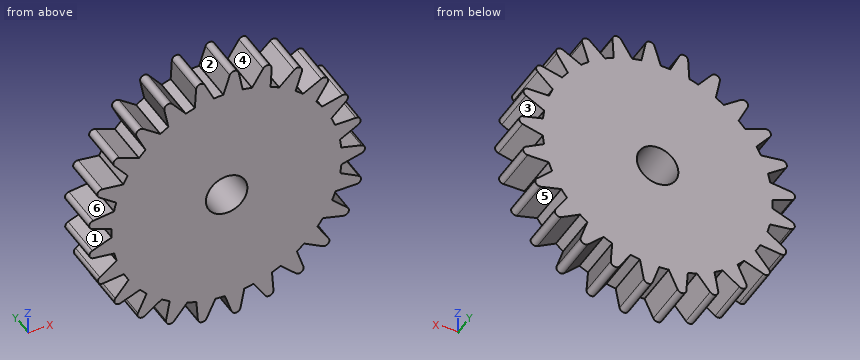
from build123d import *

# Parameters (mm, degrees)
BOSS_EXTRUDE1_DEPTH = 5
SKETCH6_R           = 2.25
CUT_EXTRUDE1_DEPTH  = 6


with BuildPart() as part:
    # Sketch1 → Boss-Extrude1 (new body)
    with BuildSketch(Plane(origin=(0, -74.1, 0), x_dir=(1, 0, 0), z_dir=(0, 1, 0))):
        with BuildLine():
            Line((-5.573417888, -7.249599077), (-3.909244984, -5.703911435))
            ThreePointArc((-3.909244984, -5.703911435), (-3.809726926, -5.099679562), (-4.369892407, -4.852263649))
            Line((-4.369892407, -4.852263649), (-6.574346511, -5.399076092))
            ThreePointArc((-6.574346511, -5.399076092), (-6.86485582, -4.975241994), (-7.172578897, -4.563735604))
            Line((-7.172578897, -4.563735604), (-5.94508593, -2.65274561))
            ThreePointArc((-5.94508593, -2.65274561), (-5.998960771, -2.042747658), (-6.603057459, -1.942412262))
            Line((-6.603057459, -1.942412262), (-8.602267858, -3.020271029))
            ThreePointArc((-8.602267858, -3.020271029), (-8.989053537, -2.681999186), (-9.389446406, -2.359948643))
            Line((-9.389446406, -2.359948643), (-8.675761274, -0.203730826))
            ThreePointArc((-8.675761274, -0.203730826), (-8.87964386, 0.37370479), (-9.489714138, 0.320655229))
            Line((-9.489714138, 0.320655229), (-11.158063091, -1.220524032))
            ThreePointArc((-11.158063091, -1.220524032), (-11.616821973, -0.989069307), (-12.084726477, -0.776710232))
            Line((-12.084726477, -0.776710232), (-11.92969264, 1.489252312))
            ThreePointArc((-11.92969264, 1.489252312), (-12.270772279, 1.997843189), (-12.848483188, 1.794741969))
            Line((-12.848483188, 1.794741969), (-14.081142194, -0.112919824))
            ThreePointArc((-14.081142194, -0.112919824), (-14.583048772, -0.00282537), (-15.089064749, 0.086498936))
            Line((-15.089064749, 0.086498936), (-15.502423555, 2.319827447))
            ThreePointArc((-15.502423555, 2.319827447), (-15.959268957, 2.72761695), (-16.468320796, 2.387225667))
            Line((-16.468320796, 2.387225667), (-17.187837357, 0.232946748))
            ThreePointArc((-17.187837357, 0.232946748), (-17.701354994, 0.214763292), (-18.213687601, 0.175440255))
            Line((-18.213687601, 0.175440255), (-19.169466196, 2.235806489))
            ThreePointArc((-19.169466196, 2.235806489), (-19.713372085, 2.517171704), (-20.121779254, 2.060878394))
            Line((-20.121779254, 2.060878394), (-20.282943498, -0.204656383))
            ThreePointArc((-20.282943498, -0.204656383), (-20.775805993, -0.349975216), (-21.262263487, -0.515474786))
            Line((-21.262263487, -0.515474786), (-22.700406786, 1.242468784))
            ThreePointArc((-22.700406786, 1.242468784), (-23.297197554, 1.379730498), (-23.57929833, 0.83620575))
            Line((-23.57929833, 0.83620575), (-23.171983715, -1.398233005))
            ThreePointArc((-23.171983715, -1.398233005), (-23.613222703, -1.661556297), (-24.043239171, -1.942833453))
            Line((-24.043239171, -1.942833453), (-25.873383342, -0.597770608))
            ThreePointArc((-25.873383342, -0.597770608), (-26.485560432, -0.613237052), (-26.623629384, -1.209841581))
            Line((-26.623629384, -1.209841581), (-25.673428985, -3.272786307))
            ThreePointArc((-25.673428985, -3.272786307), (-26.0353198, -3.637568488), (-26.381875725, -4.016949552))
            Line((-26.381875725, -4.016949552), (-28.489026078, -3.169282677))
            ThreePointArc((-28.489026078, -3.169282677), (-29.078124151, -3.336505465), (-29.063485901, -3.948702919))
            Line((-29.063485901, -3.948702919), (-27.630104303, -5.710531213))
            ThreePointArc((-27.630104303, -5.710531213), (-27.889908013, -6.153851676), (-28.131228013, -6.607498741))
            Line((-28.131228013, -6.607498741), (-30.382984542, -6.310489863))
            ThreePointArc((-30.382984542, -6.310489863), (-30.911988399, -6.618961773), (-30.745562721, -7.208285533))
            Line((-30.745562721, -7.208285533), (-28.919064562, -8.558295243))
            ThreePointArc((-28.919064562, -8.558295243), (-29.060456745, -9.052298535), (-29.181377796, -9.551707286))
            Line((-29.181377796, -9.551707286), (-31.436254358, -9.824018565))
            ThreePointArc((-31.436254358, -9.824018565), (-31.871924741, -10.254357173), (-31.564168772, -10.783777859))
            Line((-31.564168772, -10.783777859), (-29.459319649, -11.637142911))
            ThreePointArc((-29.459319649, -11.637142911), (-29.473416113, -12.150788987), (-29.466340301, -12.664579737))
            Line((-29.466340301, -12.664579737), (-31.582654708, -13.489100854))
            ThreePointArc((-31.582654708, -13.489100854), (-31.897616846, -14.014266401), (-31.467868026, -14.450518566))
            Line((-31.467868026, -14.450518566), (-29.21692335, -14.753618895))
            ThreePointArc((-29.21692335, -14.753618895), (-29.102838363, -15.254633483), (-28.968210287, -15.750522868))
            Line((-28.968210287, -15.750522868), (-30.812986722, -17.07544613))
            ThreePointArc((-30.812986722, -17.07544613), (-30.987450384, -17.662440534), (-30.462711412, -17.97811285))
            Line((-30.462711412, -17.97811285), (-28.207106316, -17.711903547))
            ThreePointArc((-28.207106316, -17.711903547), (-27.972008257, -18.168806058), (-27.718287094, -18.615635525))
            Line((-27.718287094, -18.615635525), (-29.175611469, -20.357711129))
            ThreePointArc((-29.175611469, -20.357711129), (-29.198614462, -20.969651374), (-28.611856617, -21.144908987))
            Line((-28.611856617, -21.144908987), (-26.493319064, -20.326116962))
            ThreePointArc((-26.493319064, -20.326116962), (-26.151980009, -20.710198531), (-25.795107994, -21.079892141))
            Line((-25.795107994, -21.079892141), (-26.773411257, -23.129659071))
            ThreePointArc((-26.773411257, -23.129659071), (-26.643508219, -23.728094699), (-26.031599654, -23.75192553))
            Line((-26.031599654, -23.75192553), (-24.183245151, -22.431998497))
            ThreePointArc((-24.183245151, -22.431998497), (-23.757112689, -22.719125866), (-23.319513401, -22.988454411))
            Line((-23.319513401, -22.988454411), (-23.757325162, -25.217118272))
            ThreePointArc((-23.757325162, -25.217118272), (-23.482678378, -25.764447372), (-22.88406756, -25.635354042))
            Line((-22.88406756, -25.635354042), (-21.422035016, -23.897227871))
            ThreePointArc((-21.422035016, -23.897227871), (-20.937884616, -24.069359772), (-20.44705403, -24.221400348))
            Line((-20.44705403, -24.221400348), (-20.316864965, -26.488925992))
            ThreePointArc((-20.316864965, -26.488925992), (-19.914731502, -26.950757865), (-19.367031349, -26.676851782))
            Line((-19.367031349, -26.676851782), (-18.383185648, -24.629739333))
            ThreePointArc((-18.383185648, -24.629739333), (-17.87143826, -24.676060085), (-17.358217065, -24.701259423))
            Line((-17.358217065, -24.701259423), (-16.668207433, -26.865169876))
            ThreePointArc((-16.668207433, -26.865169876), (-16.163854816, -27.212485926), (-15.701479344, -26.810977617))
            Line((-15.701479344, -26.810977617), (-15.257639128, -24.583506493))
            ThreePointArc((-15.257639128, -24.583506493), (-14.750449723, -24.501105593), (-14.247085495, -24.397880327))
            Line((-14.247085495, -24.397880327), (-13.040611138, -26.322209137))
            ThreePointArc((-13.040611138, -26.322209137), (-12.465729697, -26.533186219), (-12.117731656, -26.029303927))
            Line((-12.117731656, -26.029303927), (-12.241785039, -23.761434332))
            ThreePointArc((-12.241785039, -23.761434332), (-11.771022192, -23.555489332), (-11.309143157, -23.330325485))
            Line((-11.309143157, -23.330325485), (-9.662011296, -24.894159994))
            ThreePointArc((-9.662011296, -24.894159994), (-9.052722946, -24.955541642), (-8.840968333, -24.380946146))
            Line((-8.840968333, -24.380946146), (-9.525120585, -22.215176667))
            ThreePointArc((-9.525120585, -22.215176667), (-9.120364058, -21.898627848), (-8.728991773, -21.565673292))
            Line((-8.728991773, -21.565673292), (-6.744697761, -22.670752028))
            ThreePointArc((-6.744697761, -22.670752028), (-6.139286329, -22.578681408), (-6.077080467, -21.969476655))
            Line((-6.077080467, -21.969476655), (-7.278343785, -20.041890553))
            ThreePointArc((-7.278343785, -20.041890553), (-6.965025918, -19.634627842), (-6.668751745, -19.214803336))
            Line((-6.668751745, -19.214803336), (-4.471976071, -19.791690138))
            ThreePointArc((-4.471976071, -19.791690138), (-3.908481786, -19.551952385), (-3.999733295, -18.94641695))
            Line((-3.999733295, -18.94641695), (-5.642627888, -17.378131549))
            ThreePointArc((-5.642627888, -17.378131549), (-5.440435595, -16.905744761), (-5.257875529, -16.425429423))
            Line((-5.257875529, -16.425429423), (-2.986649689, -16.43787637))
            ThreePointArc((-2.986649689, -16.43787637), (-2.500478968, -16.065535089), (-2.739454182, -15.501716992))
            Line((-2.739454182, -15.501716992), (-4.72075094, -14.391273432))
            ThreePointArc((-4.72075094, -14.391273432), (-4.642388707, -13.883444364), (-4.585013668, -13.372818174))
            Line((-4.585013668, -13.372818174), (-2.382047135, -12.820043179))
            ThreePointArc((-2.382047135, -12.820043179), (-2.003747871, -12.338493942), (-2.375431099, -11.851819947))
            Line((-2.375431099, -11.851819947), (-4.570637859, -11.26899148))
            ThreePointArc((-4.570637859, -11.26899148), (-4.621029474, -10.757628901), (-4.692444547, -10.24877638))
            Line((-4.692444547, -10.24877638), (-2.696157809, -9.16551233))
            ThreePointArc((-2.696157809, -9.16551233), (-2.449499938, -8.605012646), (-2.930536955, -8.226062269))
            Line((-2.930536955, -8.226062269), (-5.201720804, -8.207470152))
            ThreePointArc((-5.201720804, -8.207470152), (-5.377699975, -7.724704854), (-5.573417888, -7.249599077))
        make_face()
    extrude(amount=-BOSS_EXTRUDE1_DEPTH)

    # Sketch6 → Cut-Extrude1 (cut, through all)
    with BuildSketch(Plane(origin=(0, -74.1, 0), x_dir=(1, 0, 0), z_dir=(0, 1, 0))):
        with Locations((-17.003397692, -12.235998762)):
            Circle(SKETCH6_R)
    extrude(amount=-CUT_EXTRUDE1_DEPTH, mode=Mode.SUBTRACT)


solid = part.part
Can you work these out from the model? Positions are in its coordinate system, mm. Face numbers are marked on the shaded views. A direction names the side the tool comes from. Coordinates: 2 decimals unless noted, no trailing zeros. Order: outer loops, then holes, each group sorted by start corner. A loop starts at its lowest first (then second) coordinate and runs counter-clockwise, first axis right, second up. Notation, with made-up numbers: (69, -7.75) -> (106, -7.75) arc R14 ccw to (106, 10.25) -> close; hole circle Ø2 at (17, 52). An arc over 180 degrees is marked (long way). Use one line per item in the form item = value.
Q1. Imagine slicing it at A-A, the plane x = -25.25. List the corners of the cut face in (y, z) for me, then the cut area to 3 significant figures.
From the geometry:
outline = (-79.1, 1.06) -> (-74.1, 1.06) -> (-74.1, 23.19) -> (-79.1, 23.19) -> close
area = 111 mm²
Q2. Will these pins go through, and if not, where does the flat tip stop? P1, Ø3, axis at y = -76.5, z = 20, coming from the +X side (3 decimals); P2, Ø3, axis at x = -19, y = -78, coming from the +Z side; P3, Ø3, axis at y = -75.5, z = 2, coming from the +X side.
From the geometry:
P1 = -3.845
P2 = 26.96
P3 = -5.87
Q3. Imagine slicing it at B-B, the plane x = -10.25. List the corners of the cut face in (y, z) for me.
From the geometry:
outline = (-79.1, 0.38) -> (-74.1, 0.38) -> (-74.1, 24.34) -> (-79.1, 24.34) -> close
Q4. We'd pull the mould along X, two halves only. Please class the marked faces 1, 2 and 3: released by +X, released by -X, zero draft, split by the parting line, or undercut.
From the geometry:
face_1 = released by -X
face_2 = undercut
face_3 = released by +X
Q5. I need wall thicknesses on L1, parallel to X at y = -75.7, z = 24.75; L2, parallel to X at y = -78.35, z = -1; L3, parallel to Z at x = -5.5, y = -74.25. Which ranges of each line are inside material? Lowest first, please.
From the geometry:
L1 = -23.67 to -22.14, -20.42 to -18.44, -17.34 to -15.29, -14.03 to -12.19, -9.81 to -8.87
L2 = -23.58 to -22.5, -20.2 to -18.6, -16.93 to -15.26, -13.36 to -11.96
L3 = 5.13 to 7.18, 7.42 to 17.05, 17.51 to 19.52
Q6. Which directions (+Z, -Z, +X, -X, +Y, -Y) give clear straight access to the entire face, cutting with the end or side of a thin tool? Please do the marked faces 4, 5 and 6.
From the geometry:
face_4 = +Z, +Y, -Y
face_5 = +Y, -Y
face_6 = -X, +Y, -Y
